Part print with two shaded views. Sizes in mm from the minimum x, y, z corner. A direction names the side the tool comes from. Round coordinates to 2 decimals unless told otherwise and drop trailing zeros. Loops run counter-clockwise (first coordinate to the right, second up) from the corner with the lowest first, then second, coordinate; pieces in that order, holes last. Notation, with made-up numbers: (11.5, 21) - (46.5, 21) arc R19 ccw to (46.5, 47) - close; hole circle Ø6 at (71, 81). An arc over 180 degrees is marked (long way). Write each question's results on one line, items separated by ' | '. Start each with the question number.
(1) Cut at C-C, the plane y = 24. List the corners of the cut face in (x, z).
(2) Cut at B-B, the plane x = 18.25. List the corners of the cut face in (y, z), then the cut area to 3 significant figures.
(3) Cut at D-D, the plane z = 7.75. List the corners of the cut face in (x, y).
(4) Tool access for the marked faces 1, 2, 3, 4 and 5: list every direction of +Z, -Z, +X, -X, +Y, -Y with a clear straight run to the whole face (end or side of a thin tool).
(5) Flat gauge pins, fed straight in: P1, Ø7, axis at x = 20, z = 2, coming from the +Y side; P2, Ø1.9, axis at x = 20, z = 9.5, coming from the +Y side; P3, Ø3, axis at x = 9.5, y = 25, coming from the +Z side; P4, Ø5, axis at x = 6, z = 3.5, coming from the +Y side. Where does each tip first touch, or does it go through?
(6) Drill centre lines: L1, parallel to Y at x = 7.5, z = 3.75; L2, parallel to X at y = 25.5, z = 6 (3 decimals); L3, parallel to Y at x = 10.5, z = 4.5. Where is each one in solid material? Low to high.
(7) Cut at A-A, the plane z = 2.25. List the corners of the cut face in (x, y), then the cut area to 3 significant figures.
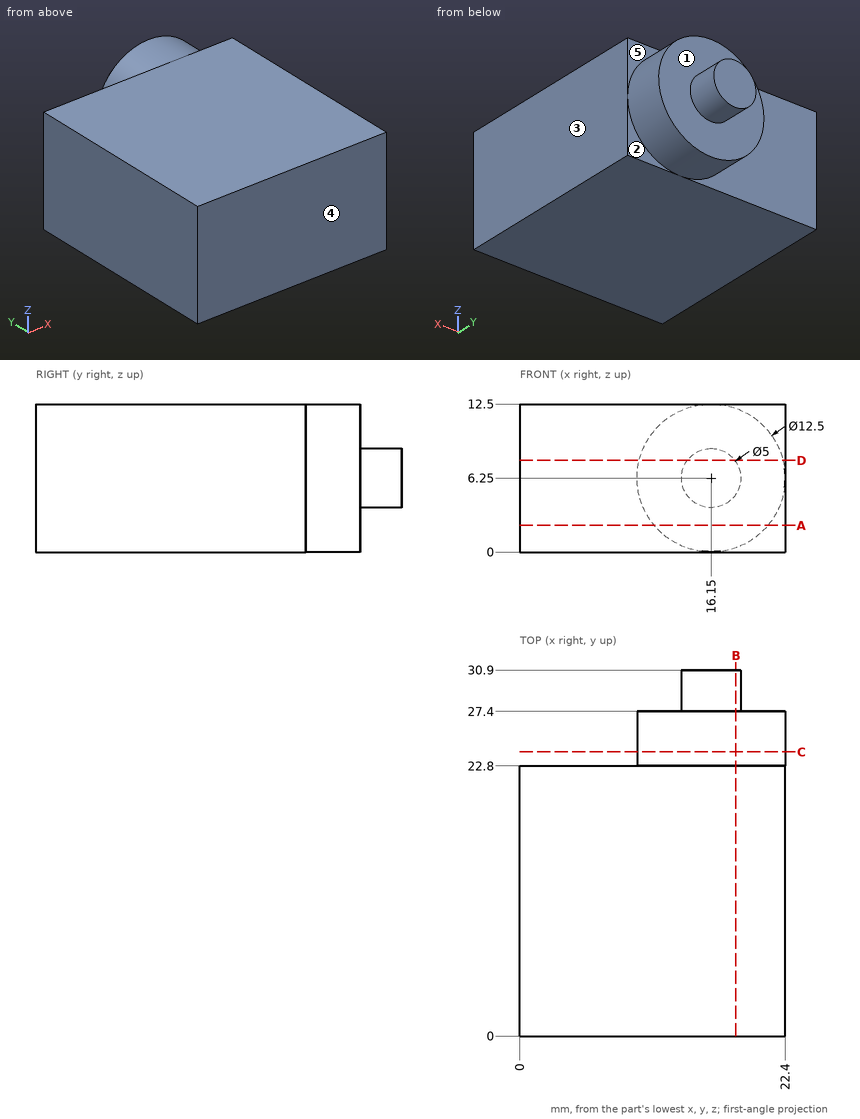
A:
1) outline: circle Ø12.5 at (16.15, 6.25)
2) outline: (0, 0) - (22.8, 0) - (22.8, 0.36) - (27.4, 0.36) - (27.4, 4.89) - (30.9, 4.89) - (30.9, 7.61) - (27.4, 7.61) - (27.4, 12.14) - (22.8, 12.14) - (22.8, 12.5) - (0, 12.5) - close | area: 349 mm2
3) outline: (0, 0) - (22.4, 0) - (22.4, 22.8) - (22.22, 22.8) - (22.22, 27.4) - (18.15, 27.4) - (18.15, 30.9) - (14.15, 30.9) - (14.15, 27.4) - (10.08, 27.4) - (10.08, 22.8) - (0, 22.8) - close
4) face 1: +Y | face 2: -Z, +X, +Y | face 3: +Z, -Z, +X, +Y, -Y | face 4: +Z, -Z, +X, -X, -Y | face 5: +Z, +X, +Y
5) P1: y = 30.9 | P2: y = 27.4 | P3: z = 9.79 | P4: y = 22.8
6) L1: 0 to 22.8 | L2: 9.905 to 22.395 | L3: 0 to 27.4
7) outline: (0, 0) - (22.4, 0) - (22.4, 22.8) - (20.95, 22.8) - (20.95, 27.4) - (11.35, 27.4) - (11.35, 22.8) - (0, 22.8) - close | area: 555 mm2
